```python
from build123d import *

# Parameters (mm, degrees)
F2_DEPTH = 1.651
F3_DEPTH = 3.175


# Not quite as in the source:
# - a feature of the source that left no trace in its solid (it failed there, or was rolled back) is left out


with BuildPart() as f2:
    # F0 (on Front) → F2 (new body)
    with BuildSketch(Plane.XZ):
        with BuildLine():
            Line((57.15, 63.5), (-57.15, 63.5))
            ThreePointArc((-57.15, 63.5), (-61.6401280605, 61.6401280605), (-63.5, 57.15))
            Line((-63.5, 57.15), (-63.5, -57.15))
            ThreePointArc((-63.5, -57.15), (-61.6401280605, -61.6401280605), (-57.15, -63.5))
            Line((-57.15, -63.5), (57.15, -63.5))
            ThreePointArc((57.15, -63.5), (61.6401280605, -61.6401280605), (63.5, -57.15))
            Line((63.5, -57.15), (63.5, 57.15))
            ThreePointArc((63.5, 57.15), (61.6401280605, 61.6401280605), (57.15, 63.5))
        make_face()
    extrude(amount=F2_DEPTH)

    # F1 (on face) → F3 (join)
    with BuildSketch(Plane.XZ):
        with BuildLine():
            Line((58.928, 65.278), (-58.928, 65.278))
            ThreePointArc((-58.928, 65.278), (-63.4181280605, 63.4181280605), (-65.278, 58.928))
            Line((-65.278, 58.928), (-65.278, -58.928))
            ThreePointArc((-65.278, -58.928), (-63.4181280605, -63.4181280605), (-58.928, -65.278))
            Line((-58.928, -65.278), (58.928, -65.278))
            ThreePointArc((58.928, -65.278), (63.4181280605, -63.4181280605), (65.278, -58.928))
            Line((65.278, -58.928), (65.278, 58.928))
            ThreePointArc((65.278, 58.928), (63.4181280605, 63.4181280605), (58.928, 65.278))
        make_face()
        with BuildLine():
            ThreePointArc((29.1683860123, 0), (21.2359008795, -15.4304684341), (4.5518055526, -20.1912078303))
            ThreePointArc((4.5518055526, -20.1912078303), (12.5076591177, -4.7892295638), (29.1683860123, 0))
        make_face(mode=Mode.SUBTRACT)
        with BuildLine():
            ThreePointArc((-30.0225467432, 26.633475086), (-11.3001914874, 17.269662026), (-5.1093608776, -2.7273676961))
            ThreePointArc((-5.1093608776, -2.7273676961), (-23.8921161087, 6.5851949341), (-30.0225467432, 26.633475086))
        make_face(mode=Mode.SUBTRACT)
        with BuildLine():
            Line((-5.3865113296, -11.8381703437), (-5.3865113296, -57.15))
            Line((-5.3865113296, -57.15), (-50.8, -57.15))
            ThreePointArc((-50.8, -57.15), (-55.2901280605, -55.2901280605), (-57.15, -50.8))
            Line((-57.15, -50.8), (-57.15, 50.8))
            ThreePointArc((-57.15, 50.8), (-55.2901280605, 55.2901280605), (-50.8, 57.15))
            Line((-50.8, 57.15), (50.8, 57.15))
            ThreePointArc((50.8, 57.15), (55.2901280605, 55.2901280605), (57.15, 50.8))
            Line((57.15, 50.8), (57.15, -50.8))
            ThreePointArc((57.15, -50.8), (55.2901280605, -55.2901280605), (50.8, -57.15))
            Line((50.8, -57.15), (2.8426104691, -57.15))
            Line((2.8426104691, -57.15), (2.8426104691, -28.5558674872))
            ThreePointArc((2.8426104691, -28.5558674872), (29.0723668952, -19.260680993), (37.6052677218, 7.2268673576))
            ThreePointArc((37.6052677218, 7.2268673576), (18.8257654598, 7.524261984), (3.0884773301, -2.7273676961))
            ThreePointArc((3.0884773301, -2.7273676961), (-7.830876963, 25.422268659), (-36.6427004337, 34.4507321715))
            ThreePointArc((-36.6427004337, 34.4507321715), (-32.213387286, 3.7443986853), (-5.3865113296, -11.8381703437))
        make_face(mode=Mode.SUBTRACT)
    extrude(amount=F3_DEPTH)


solid = f2.part
```
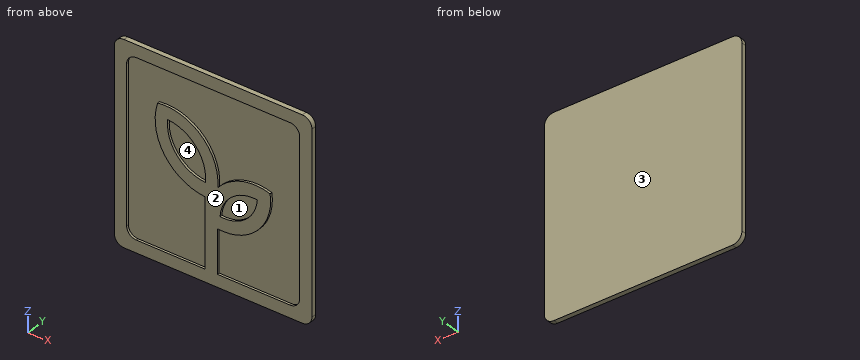
Input: part model. Units: mm. Frame: model coordinates. Face numbers are marked on the shaded views. A direction names the side the tool comes from. Give positions to 0.01 mm unless a question says otherwise; leave off trailing zeros. Order: outer loops, then holes, each group sorted by start corner. A loop starts at its lowest first (then second) coordinate and runs counter-clockwise, first axis right, second up.
1. Pin query (flat end, axial travel): pin 1 (7.5 mm diameter, centred on x = -18.5, z = 17, fed in from -Y). Return the tip coordinate at first contact, or that it passes through.
Derived:
pin 1: stops at y = -1.65
2. Section B-B on x = 42. Return the cut outline in (y, z) (3 decimals), and give its area (3 significant figures).
Derived:
outline: (-3.175, -65.278) - (0, -65.278) - (0, 65.278) - (-3.175, 65.278) - (-3.175, 57.15) - (-1.651, 57.15) - (-1.651, -57.15) - (-3.175, -57.15) - close
area: 240 mm2
3. Section A-A on z = -45. Return the cut outline in (x, y) (3 decimals), and give its area (3 significant figures).
Derived:
outline: (-65.278, -3.175) - (-57.15, -3.175) - (-57.15, -1.651) - (-5.387, -1.651) - (-5.387, -3.175) - (2.843, -3.175) - (2.843, -1.651) - (57.15, -1.651) - (57.15, -3.175) - (65.278, -3.175) - (65.278, 0) - (-65.278, 0) - close
area: 253 mm2
4. Reachability of the marked faces 1 and 2 from +Z, -Z, +X, -X, +Y, -Y: full face, straight path, thin tool, end or side. Return the list, or none.
Derived:
face 1: -Y
face 2: +Z, -Z, +X, -X, -Y
5. Material intervals for L1, parallel to Z at x = -38.5, y = -2.65; L2, parallel to X at y = -2.5, z = 20; L3, parallel to Z at x = 16.5, y = -1.7, sorted ascending.
Derived:
L1: z = -65.28 to -57.15, 57.15 to 65.28
L2: x = -65.28 to -57.15, -38.12 to -29.92, -13.98 to -3.12, 57.15 to 65.28
L3: z = -65.28 to -57.15, -27.16 to -18.39, -2.19 to 6.76, 57.15 to 65.28
6. Section C-C on x = 17. Return the cut outline in (y, z) (3 decimals).
Derived:
outline: (-3.175, -65.278) - (0, -65.278) - (0, 65.278) - (-3.175, 65.278) - (-3.175, 57.15) - (-1.651, 57.15) - (-1.651, 6.938) - (-3.175, 6.938) - (-3.175, -1.94) - (-1.651, -1.94) - (-1.651, -18.153) - (-3.175, -18.153) - (-3.175, -26.99) - (-1.651, -26.99) - (-1.651, -57.15) - (-3.175, -57.15) - close
7. Section D-D on z = -10. Return the cut outline in (x, y) (3 decimals).
Derived:
outline: (-65.278, -3.175) - (-57.15, -3.175) - (-57.15, -1.651) - (-14.291, -1.651) - (-14.291, -3.175) - (7.898, -3.175) - (7.898, -1.651) - (25.978, -1.651) - (25.978, -3.175) - (35.302, -3.175) - (35.302, -1.651) - (57.15, -1.651) - (57.15, -3.175) - (65.278, -3.175) - (65.278, 0) - (-65.278, 0) - close
8. Mould query, pull axis X, two halves, no side actions, for the marked faces 3 and 4. Classes: released by +X, released by -X, zero draft, split by the parting line, or undercut.
Derived:
face 3: zero draft
face 4: undercut
